Verification items for the finished model (mm, model axes). A direction names the side the tool comes from. Round coordinates to 2 decimals unless told otherwise and drop trailing zeros. Order: outer loops, then holes, each group sorted by start corner. A loop starts at its lowest first (then second) coordinate and runs counter-clockwise, first axis right, second up. Notation, with made-up numbers: (31.25, 8) -> (83.25, 8) arc R14 cw to (83.25, 17) -> close; hole circle Ø4 at (77, 1). An arc over 180 degrees is marked (long way). Return JSON: item names as keys, results as strings. Group by question number.
Item 1: Sectioned sample at A-A on x = 1. Record the cut outline in (y, z).
Item 2: Sectioned sample at C-C on y = 1.5. Record the cut outline in (x, z), plus the area to 3 significant figures.
Item 3: Depth check by flat-ended pin: pin 1 Ø1 at (x, z) = (7, 2.5) entering from -Y; pin 2 Ø2 at (x, z) = (1.5, 2.5) entering from -Y; pin 3 Ø1.2 at (x, y) = (13.5, 4) entering from -Z. Enter the tip coordinate at first touch or a pass-through.
Item 4: Scan lines: probe 1 along Z at (x, y) = (24.5, 3.75); probe 2 along Y at (x, z) = (3, -0.25); probe 3 along Z at (x, y) = (28, 2.75). Record each from-to range of solid material in increasing order. Write a range as from..to.
Item 5: Sectioned sample at B-B on z = -2. Record the cut outline in (x, y), plus the area to 3 significant figures.
Item 6: Sectioned sample at D-D on y = -1.25. Record the cut outline in (x, z), plus the area to 3 significant figures.
Item 7: Access from +Z, -Z, +X, -X, +Y, -Y to the whole of each face (thin tool, end or side, straight path). Record for faces 1 (the flat face through (13, 4, 1.5)), 2 (the flat face through (-10, 1, 0)), 3 (the flat face through (13, 4, -1.5)).
```python
from build123d import *
from build123d.topology import SkipClean

# Parameters (mm, degrees)
BOSS_EXTRU_1_DEPTH           = 50
ENL_V_START                  = -6
ENL_V_MAT_EXTRU_1_DEPTH      = 6
ESQUISSE5_R                  = 3.5
BOSS_EXTRU_2_DEPTH           = 10
ENL_V_MAT_EXTRU_2_DEPTH      = 10
ENL_V_MAT_EXTRU_2_DEPTH_BACK = 10
ESQUISSE6_W                  = 18.121424082
ESQUISSE6_H                  = 16.818170981
BOSS_EXTRU_3_DEPTH           = 16


with BuildPart() as part:
    # Esquisse1 → Boss.-Extru.1 (new body)
    with BuildSketch(Plane(origin=(0, 0, 0), x_dir=(0, 0, -1), z_dir=(1, 0, 0))):
        with BuildLine():
            ThreePointArc((1.5, 3.16227766), (0, 3.5), (-1.5, 3.16227766))
            Line((-1.5, 3.16227766), (1.5, 3.16227766))
        make_face()
        with BuildLine():
            Line((1.5, 3.16227766), (-1.5, 3.16227766))
            ThreePointArc((-1.5, 3.16227766), (-1.870828693, -2.958039892), (3.5, 0))
            ThreePointArc((3.5, 0), (2.958039892, 1.870828693), (1.5, 3.16227766))
        make_face()
        with BuildLine():
            Line((-1.5, 4.66227766), (-1.5, 3.16227766))
            ThreePointArc((-1.5, 3.16227766), (0, 3.5), (1.5, 3.16227766))
            Line((1.5, 3.16227766), (1.5, 4.66227766))
            Line((1.5, 4.66227766), (-1.5, 4.66227766))
        make_face()
    extrude(amount=BOSS_EXTRU_1_DEPTH)

    # Esquisse4 → Enlèv. mat.-Extru.1 (cut)
    with BuildSketch(Plane(origin=(50, 0, 0), x_dir=(0, 0, -1), z_dir=(1, 0, 0)).offset(ENL_V_START)):
        with BuildLine():
            Line((-1.5, 3.16227766), (-1.5, 4.66227766))
            Line((-1.5, 4.66227766), (1.5, 4.66227766))
            Line((1.5, 4.66227766), (1.5, 3.16227766))
            ThreePointArc((1.5, 3.16227766), (0, 3.5), (-1.5, 3.16227766))
        make_face()
    enl_v_mat_extru_1 = extrude(amount=ENL_V_MAT_EXTRU_1_DEPTH, mode=Mode.SUBTRACT)

    # Symétrie1: Enlèv. mat.-Extru.1 across plane
    with SkipClean():  # the faces are left unmerged after this step: merging them gives an invalid solid
        add(enl_v_mat_extru_1.mirror(Plane(origin=(25, 0, 0), x_dir=(0, 0, 1), z_dir=(1, 0, 0))), mode=Mode.SUBTRACT)

    # Esquisse5 → Boss.-Extru.2 (add)
    with SkipClean():  # the faces are left unmerged after this step: merging them gives an invalid solid
        with BuildSketch(Plane.ZY):
            Circle(ESQUISSE5_R)
        extrude(amount=BOSS_EXTRU_2_DEPTH)

    # Esquisse6 → Enlèv. mat.-Extru.2 (cut, two sides: drawn at the far end of the back side and taken through both)
    with SkipClean():  # the faces are left unmerged after this step: merging them gives an invalid solid
        with BuildSketch(Plane.XY.offset(-ENL_V_MAT_EXTRU_2_DEPTH_BACK)):
            with Locations((43.560712041, -0.183428049)):
                Rectangle(ESQUISSE6_W, ESQUISSE6_H)
        extrude(amount=ENL_V_MAT_EXTRU_2_DEPTH + ENL_V_MAT_EXTRU_2_DEPTH_BACK, mode=Mode.SUBTRACT)

    # Esquisse8 → Boss.-Extru.3 (add)
    with BuildSketch(Plane.ZY.offset(-6)):
        with BuildLine():
            Line((1.5, 3.16227766), (1.5, 4.66227766))
            Line((1.5, 4.66227766), (-1.5, 4.66227766))
            Line((-1.5, 4.66227766), (-1.5, 3.16227766))
            ThreePointArc((-1.5, 3.16227766), (0, 3.5), (1.5, 3.16227766))
        make_face()
    extrude(amount=BOSS_EXTRU_3_DEPTH)


solid = part.part
```
Recorded:
{
 "1": {"outline": "(3.16, -1.5) -> (4.66, -1.5) -> (4.66, 1.5) -> (3.16, 1.5) arc R3.5 ccw (long way) to start"},
 "2": {"outline": "(-10, -3.16) -> (34.5, -3.16) -> (34.5, 3.16) -> (-10, 3.16) -> close", "area": "281 mm²"},
 "3": {"pin 1": "y = -2.87", "pin 2": "y = -3.16", "pin 3": "z = -1.5"},
 "4": {"probe 1": "-1.5..1.5", "probe 2": "-3.49..4.66", "probe 3": "-2.17..2.17"},
 "5": {"outline": "(-10, -2.87) -> (34.5, -2.87) -> (34.5, 2.87) -> (-10, 2.87) -> close", "area": "256 mm²"},
 "6": {"outline": "(-10, -3.27) -> (34.5, -3.27) -> (34.5, 3.27) -> (-10, 3.27) -> close", "area": "291 mm²"},
 "7": {"face 1": "+Z, +X, -X, +Y", "face 2": "+Z, -Z, -X, +Y, -Y", "face 3": "-Z, +X, -X, +Y"}
}
